Here's how the part is built. I have some questions about the finished solid (model axes, mm). A direction names the side the tool comes from. Round coordinates to 2 decimals unless told otherwise and drop trailing zeros. Loops run counter-clockwise (first coordinate to the right, second up) from the corner with the lowest first, then second, coordinate; pieces in that order, holes last. Notation, with made-up numbers: M -13,-24.5 L 23,-24.5 A20 cw 23,0.5 Z; hole C -28,35.25 d4. An arc over 180 degrees is marked long. Answer as a JSON object with one key per item and string values.
from build123d import *

# Parameters (mm, degrees)
SKETCH1_R           = 15.24
SKETCH1_R_2         = 12.7
BOSS_EXTRUDE1_DEPTH = 38.1
SKETCH2_R           = 0.9525
CUT_EXTRUDE1_DEPTH  = 5.08


with BuildPart() as part:
    # Sketch1 → Boss-Extrude1 (new body)
    with BuildSketch(Plane(origin=(0, 0, 0), x_dir=(1, 0, 0), z_dir=(0, 1, 0))):
        with Locations(Location((0, 0, 0), (0, 0, 90))):
            Circle(SKETCH1_R)
        with Locations(Location((0, 0, 0), (0, 0, 90))):
            Circle(SKETCH1_R_2, mode=Mode.SUBTRACT)
    extrude(amount=BOSS_EXTRUDE1_DEPTH)

    # Sketch2 → Cut-Extrude1 (cut)
    with BuildSketch(Plane(origin=(0, 38.1, 0), x_dir=(1, 0, 0), z_dir=(0, 1, 0))):
        with Locations(Location((-13.97, 0, 0), (0, 0, 270))):
            Circle(SKETCH2_R)
        with Locations(Location((13.97, 0, 0), (0, 0, 270))):
            Circle(SKETCH2_R)
    extrude(amount=-CUT_EXTRUDE1_DEPTH, mode=Mode.SUBTRACT)


solid = part.part
Item 1: I want a section at C-C on y = 18. List the corners of the cut face in (x, z) for me.
Solution:
{"outline": "C 0,0 d30.48; hole C 0,0 d25.4"}
Item 2: I want a section at D-D on x = -13.97. List the corners of the cut face in (y, z) for me, plus the area to 3 significant figures.
Solution:
{"outline": "M 0,-6.09 L 38.1,-6.09 L 38.1,-0.95 L 33.02,-0.95 L 33.02,0.95 L 38.1,0.95 L 38.1,6.09 L 0,6.09 Z", "area": "454 mm2"}
Item 3: For P1, Ø4, axis at x = 8, y = 31.5, coming from the +Z side; P2, Ø1, axis at y = 26.5, z = -2.5, coming from the +X side; P3, Ø5, axis at y = 16, z = -9, coming from the +X side; P4, Ø1, axis at x = -1.5, z = 11, coming from the +Y side, each with a flat end and sliding along its axis, tell me the tip position at first contact or that it passes through.
Solution:
{"P1": "stops at z = 14.01", "P2": "stops at x = 15.11", "P3": "stops at x = 13.78", "P4": "passes through"}
Item 4: We'd pull the mould along Z, two halves only. Please class faces 3 (the face through (-12.5, 0, 3.5)), 4 (the face through (-15.11, 18.78, 1.98)), 5 (the face through (14.914, 35.596, -0.124)): +Z half, -Z half, draft (parallel to the pull), parting line (faces both ways), or undercut.
Solution:
{"face 3": "draft", "face 4": "parting line", "face 5": "undercut"}
Item 5: I want a section at A-A on z = 0. List the corners of the cut face in (x, y) for me.
Solution:
{"outline": "M -15.24,0 L -12.7,0 L -12.7,38.1 L -13.02,38.1 L -13.02,33.02 L -14.92,33.02 L -14.92,38.1 L -15.24,38.1 Z; M 12.7,0 L 15.24,0 L 15.24,38.1 L 14.92,38.1 L 14.92,33.02 L 13.02,33.02 L 13.02,38.1 L 12.7,38.1 Z"}
Item 6: I want a section at B-B on x = 0. List the corners of the cut face in (y, z) for me.
Solution:
{"outline": "M 0,-15.24 L 38.1,-15.24 L 38.1,-12.7 L 0,-12.7 Z; M 0,12.7 L 38.1,12.7 L 38.1,15.24 L 0,15.24 Z"}
Item 7: For faces 1 (the face through (14, 33.02, 0)), 2 (the face through (7.7, 18.8, 10.1)), which set-ups out of +Z, -Z, +X, -X, +Y, -Y let a thin tool reach every point of the face, with its end or its side?
Solution:
{"face 1": "+Y", "face 2": "+Y, -Y"}
Item 8: If I drill on L1, parallel to X at y = 36, z = 0; L2, parallel to X at y = 24, z = 0; L3, parallel to Z at x = -10, y = 20.5, over which ranges is the centre line in solid material (lowest first)? Write a range as from..to.
Solution:
{"L1": "x = -15.24..-14.92, -13.02..-12.7, 12.7..13.02, 14.92..15.24", "L2": "x = -15.24..-12.7, 12.7..15.24", "L3": "z = -11.5..-7.83, 7.83..11.5"}
